Part model, mm, in its own coordinate system. Face numbers are marked on the shaded views. A direction names the side the tool comes from. Coordinates: 2 decimals unless noted, no trailing zeros. Order: outer loops, then holes, each group sorted by start corner. A loop starts at its lowest first (then second) coordinate and runs counter-clockwise, first axis right, second up.
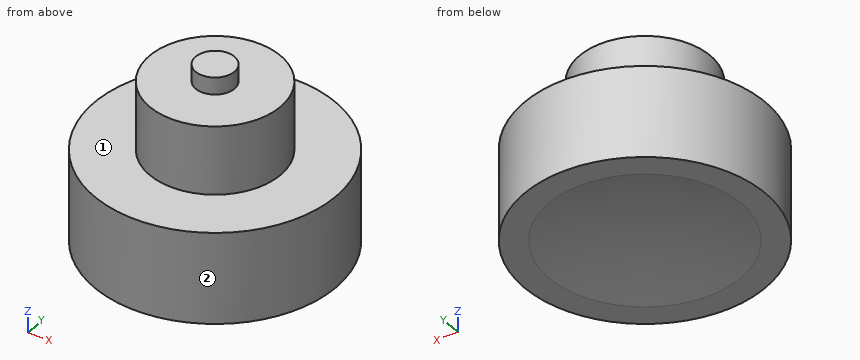
from build123d import *


with BuildPart() as part:
    # Sketch1 → Revolve1 (revolve)
    with BuildSketch(Plane(origin=(0, 0, 0), x_dir=(0, 0, -1), z_dir=(1, 0, 0)), mode=Mode.PRIVATE) as revolve1_sk:
        Polygon((0, 0), (-65.659, 0), (-65.659, 7.182450088), (-59.309, 7.182450088), (-59.309, 24.257), (-33.909, 24.257), (-33.909, 44.704), (0, 44.704), align=None)
    revolve(revolve1_sk.sketch.rotate(Axis((0, 0, 0), (0, 0, -1)), 90), axis=Axis((0, 0, 0), (0, 0, -1)))

    # Sketch2 → Cut-Revolve5 (revolve, cut)
    with BuildSketch(Plane(origin=(0, 0, 0), x_dir=(0, 0, -1), z_dir=(1, 0, 0))):
        with BuildLine():
            Line((-5.08, 0), (248.92, 0))
            ThreePointArc((248.92, 0), (121.92, 127), (-5.08, 0))
        make_face()
    revolve(axis=Axis((0, 0, 5.08), (0, 0, -1)), mode=Mode.SUBTRACT)


solid = part.part
Q1. Cut at B-B on y = 12. Write the cut outline in (x, z).
Results list:
outline: (-43.06, 0) - (-33.47, 0) arc R126.43 cw to (33.47, 0) - (43.06, 0) - (43.06, 33.91) - (21.08, 33.91) - (21.08, 59.31) - (-21.08, 59.31) - (-21.08, 33.91) - (-43.06, 33.91) - close
Q2. Cut at C-C on z = 21. Write the cut outline in (x, y).
Results list:
outline: circle Ø89.41 at (0, 0)
Q3. Pin check, flat tips, straight feed: pin 1 Ø10 at (y, z) = (22, 10.5) entering from +X; pin 2 Ø12 at (y, z) = (-27, 46) entering from +X; pin 3 Ø5 at (y, z) = (8.5, 18) entering from +X. Stop position of each tip, or through.
Results list:
pin 1: stops at x = 41.35
pin 2: stops at x = 12.14
pin 3: stops at x = 44.3
Q4. Wall check: line 1 along Z through (x, y) = (-32, 26.5); line 2 along X through (y, z) = (-34, 24.5); line 3 along X through (y, z) = (-15.5, 14.5). Give the ranges that are in metal, low to high.
Results list:
line 1: z = 0 to 33.91
line 2: x = -29.02 to 29.02
line 3: x = -41.93 to 41.93
Q5. Cut at A-A on x = 0. Write the cut outline in (y, z).
Results list:
outline: (-44.7, 0) - (-35.56, 0) arc R127 cw to (35.56, 0) - (44.7, 0) - (44.7, 33.91) - (24.26, 33.91) - (24.26, 59.31) - (7.18, 59.31) - (7.18, 65.66) - (-7.18, 65.66) - (-7.18, 59.31) - (-24.26, 59.31) - (-24.26, 33.91) - (-44.7, 33.91) - close
Q6. Which spindle directions (+Z, -Z, +X, -X, +Y, -Y) get a long thin tool onto all of the face, cutting with end or side? Do the marked faces 1 and 2. Say none if no direction does.
Results list:
face 1: +Z
face 2: +Z, -Z
